```python
from build123d import *

# Parameters (mm, degrees)
F2_DEPTH = 1.75
F3_R     = 2
F4_DEPTH = 3.501


with BuildPart() as f2:
    # F1 (on Top) → F2 (new body, symmetric)
    with BuildSketch(Plane.XY):
        Polygon((-18.75, 5.700945), (-18.75, 0), (-18.75, -4.819782), (-16.109731, -4.819782), (-16.109731, -7.483373), (-13.283064, -7.483373), (-13.283064, -10.255682), (-9.499629, -10.255682), (-9.499629, -14.045903), (-5.477123, -14.045903), (-5.477123, -17.519886), (-2.094561, -17.519886), (-2.094561, -21.176709), (0, -21.176709), (2.094561, -21.176709), (2.094561, -17.519886), (5.477123, -17.519886), (5.477123, -14.045903), (9.499629, -14.045903), (9.499629, -10.255682), (13.283064, -10.255682), (13.283064, -7.483373), (16.109731, -7.483373), (16.109731, -4.819782), (18.75, -4.819782), (18.75, 0), (18.75, 5.700945), (14.710603, 5.700945), (14.710603, 9.496642), (6.117067, 9.496642), (6.117067, 5.792365), (2.551664, 5.792365), (2.551664, 1.9527), (0, 1.9527), (-2.551664, 1.9527), (-2.551664, 5.792365), (-6.117067, 5.792365), (-6.117067, 9.496642), (-14.710603, 9.496642), (-14.710603, 5.700945), align=None)
    extrude(amount=F2_DEPTH, both=True)

    # F3 (on face) → F4 (cut, through all)
    with BuildSketch(Plane.XY.offset(1.75)):
        with Locations((-11.519544, 1.989414)):
            Circle(F3_R)
    extrude(amount=-F4_DEPTH, mode=Mode.SUBTRACT)


solid = f2.part
```
Source: CAD feature listing. Evaluate the final solid. Frame: model axes, mm. A direction names the side the tool comes from. Round coordinates to 2 decimals unless told otherwise and drop trailing zeros. Loops run counter-clockwise (first coordinate to the right, second up) from the corner with the lowest first, then second, coordinate; pieces in that order, holes last. Notation, with made-up numbers: M -0.75,68.25 L 14.25,68.25 A34 ccw 14.25,99.25 Z; hole C 86,-35 d11. An arc over 180 degrees is marked long. Use a Markdown table: item, result. Add a question column.
1. Section query D-D on y = 1. Return the cut outline in (x, z), then the cut area to 3 significant figures.
2. Section query A-A on y = 5. Return the cut outline in (x, z).
3. Section query C-C on y = -15.5. Return the cut outline in (x, z), then the cut area to 3 significant figures.
4. Section query B-B on x = 10. Return the cut outline in (y, z).
5. Mould query, pull axis X, two halves, no side actions, for faces 6 (the flat face through (-2.552, 4, 0)), 7 (the flat face through (18.75, 0, 0)), 8 (the flat face through (-13.283, -9, 0)). Classes: pulls with the +X half, pulls with the -X half, needs draft (parallel to the pull), parting line crosses it, or undercut.
6. Contact query for flat-ended pins moving along their axis: P1, Ø2.5, axis at x = -11.52, y = 1.99, coming from the -Z side (1 decimal); P2, Ø1.8, axis at y = 7, z = 0, coming from the -X side; P3, Ø1, axis at x = -1, z = 0, coming from the +Y side. Output: stop coordinate, or through.
7. Line query: line 1 (X direction, y = 7.5, z = -0.9); line 2 (Y direction, x = 13, z = -1.1); line 3 (Y direction, x = -6, z = 0.45). Output: solid intervals per line, ascending.
8. Reachability of faces 1 (the flat face through (17, 5.701, 0)), 2 (the flat face through (-6.117, 8, 0)), 3 (the flat face through (2.095, -19, 0)), 4 (the flat face through (-5.477, -16, 0)), 5 (the flat face through (-17, 5.701, 0)) from +Z, -Z, +X, -X, +Y, -Y: full face, straight path, thin tool, end or side. Return the list, or none.
Reported:
| question | item | result |
|---|---|---|
| 1 | outline | M -18.75,-1.75 L -13.26,-1.75 L -13.26,1.75 L -18.75,1.75 Z; M -9.78,-1.75 L 18.75,-1.75 L 18.75,1.75 L -9.78,1.75 Z |
| 1 | area | 119 mm² |
| 2 | outline | M -18.75,-1.75 L -2.55,-1.75 L -2.55,1.75 L -18.75,1.75 Z; M 2.55,-1.75 L 18.75,-1.75 L 18.75,1.75 L 2.55,1.75 Z |
| 3 | outline | M -5.48,-1.75 L 5.48,-1.75 L 5.48,1.75 L -5.48,1.75 Z |
| 3 | area | 38.3 mm² |
| 4 | outline | M -10.26,-1.75 L 9.5,-1.75 L 9.5,1.75 L -10.26,1.75 Z |
| 5 | face 6 | undercut |
| 5 | face 7 | pulls with the +X half |
| 5 | face 8 | pulls with the -X half |
| 6 | P1 | passes through |
| 6 | P2 | stops at x = -14.71 |
| 6 | P3 | stops at y = 1.95 |
| 7 | line 1 | x = -14.71 to -6.12, 6.12 to 14.71 |
| 7 | line 2 | y = -10.26 to 9.5 |
| 7 | line 3 | y = -14.05 to 5.79 |
| 8 | face 1 | +Z, -Z, +X, +Y |
| 8 | face 2 | +Z, -Z, +Y |
| 8 | face 3 | +Z, -Z, +X, -Y |
| 8 | face 4 | +Z, -Z, -X, -Y |
| 8 | face 5 | +Z, -Z, -X, +Y |
